The model under review builds one solid part; all positions refer to its coordinate system, in mm. Coordinates: 2 decimals unless noted, no trailing zeros. Order: outer loops, then holes, each group sorted by start corner. A loop starts at its lowest first (then second) coordinate and runs counter-clockwise, first axis right, second up.
```python
from build123d import *

# Parameters (mm, degrees)
BOSS_EXTRUDE1_DEPTH = 2
CUT_EXTRUDE1_DEPTH  = 56.375536238


with BuildPart() as part:
    # Sketch1 → Boss-Extrude1 (new body)
    with BuildSketch(Plane(origin=(0, 0, 0), x_dir=(0, 0, -1), z_dir=(1, 0, 0))):
        with BuildLine():
            Line((0, 9.101653344), (0, 0))
            Line((0, 0), (54, 0))
            Line((54, 0), (54, 1))
            Line((54, 1), (50.535898385, 3))
            Line((50.535898385, 3), (32.535898385, 3))
            Line((32.535898385, 3), (32.535898385, 5))
            Line((32.535898385, 5), (28, 5))
            Line((28, 5), (28, 8.117217781))
            ThreePointArc((28, 8.117217781), (27.749678176, 8.779020345), (27.124034735, 9.109495658))
            Line((27.124034735, 9.109495658), (3.372104204, 12.078486975))
            ThreePointArc((3.372104204, 12.078486975), (1.01459231, 11.350687872), (0, 9.101653344))
        make_face()
        with BuildLine():
            Line((0, 0), (0, -9.101653344))
            ThreePointArc((0, -9.101653344), (1.01459231, -11.350687872), (3.372104204, -12.078486975))
            Line((3.372104204, -12.078486975), (27.124034735, -9.109495658))
            ThreePointArc((27.124034735, -9.109495658), (27.749678176, -8.779020345), (28, -8.117217781))
            Line((28, -8.117217781), (28, -5))
            Line((28, -5), (32.535898385, -5))
            Line((32.535898385, -5), (32.535898385, -3))
            Line((32.535898385, -3), (50.535898385, -3))
            Line((50.535898385, -3), (54, -1))
            Line((54, -1), (54, 0))
            Line((54, 0), (0, 0))
        make_face()
    extrude(amount=BOSS_EXTRUDE1_DEPTH)

    # Sketch2 → Cut-Extrude1 (cut, through all)
    with BuildSketch(Plane(origin=(2, 0, 0), x_dir=(0, 0, -1), z_dir=(1, 0, 0))):
        with BuildLine():
            Line((4.5, -7.578486975), (3.5, -7.578486975))
            ThreePointArc((3.5, -7.578486975), (2.792893219, -7.285593756), (2.5, -6.578486975))
            Line((2.5, -6.578486975), (2.5, 6.421513025))
            ThreePointArc((2.5, 6.421513025), (2.792893219, 7.128619807), (3.5, 7.421513025))
            Line((3.5, 7.421513025), (4.5, 7.421513025))
            ThreePointArc((4.5, 7.421513025), (5.207106781, 7.128619807), (5.5, 6.421513025))
            Line((5.5, 6.421513025), (5.5, -6.578486975))
            ThreePointArc((5.5, -6.578486975), (5.207106781, -7.285593756), (4.5, -7.578486975))
        make_face()
    extrude(amount=-CUT_EXTRUDE1_DEPTH, mode=Mode.SUBTRACT)


solid = part.part
```
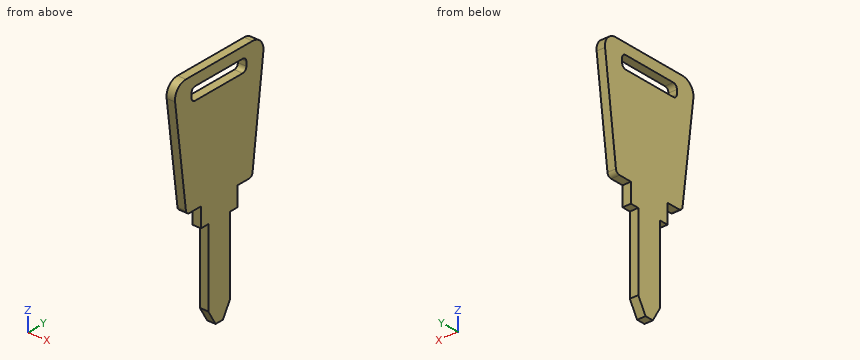
(1) We need section B-B, the plane x = 0.3. Write out the cut boundary in (y, z).
A:
outline: (-12.08, -3.37) - (-9.11, -27.12) arc R1 ccw to (-8.12, -28) - (-5, -28) - (-5, -32.54) - (-3, -32.54) - (-3, -50.54) - (-1, -54) - (1, -54) - (3, -50.54) - (3, -32.54) - (5, -32.54) - (5, -28) - (8.12, -28) arc R1 ccw to (9.11, -27.12) - (12.08, -3.37) arc R3 ccw to (9.1, 0) - (-9.1, 0) arc R3 ccw to start; hole (-7.58, -4.5) arc R1 ccw to (-6.58, -5.5) - (6.42, -5.5) arc R1 ccw to (7.42, -4.5) - (7.42, -3.5) arc R1 ccw to (6.42, -2.5) - (-6.58, -2.5) arc R1 ccw to (-7.58, -3.5) - close
(2) We need section D-D, the plane z = -6. Write out the cut boundary in (x, y).
A:
outline: (0, -11.75) - (2, -11.75) - (2, 11.75) - (0, 11.75) - close
(3) Wall thickness on probe 1 along Z at (x, y) = (1.8, 0); probe 2 along Z at (x, y) = (0.25, -4.25); probe 3 along Y at (x, z) = (1.25, -29): over which ranges is each line inside the solid? List them lowest first.
A:
probe 1: z = -54 to -5.5, -2.5 to 0
probe 2: z = -32.54 to -5.5, -2.5 to 0
probe 3: y = -5 to 5
(4) We need section A-A, the plane y = 4.25. Write out the cut boundary in (x, z), and give its area (3 significant figures).
A:
outline: (0, -32.54) - (2, -32.54) - (2, -5.5) - (0, -5.5) - close; (0, -2.5) - (2, -2.5) - (2, 0) - (0, 0) - close
area: 59.1 mm2
(5) For pin 1 Ø0.6 at (x, y) = (1, 6) entering from -Z; pin 2 Ø0.6 at (x, y) = (1.5, -3) entering from -Z; pin 3 Ø2 at (y, z) = (3.5, -10.5) entering from -X; pin 4 Ø0.6 at (x, z) = (1.5, -38.5) entering from -Y, all flat-tipped, find the tip position at first contact; note any pin that passes through.
A:
pin 1: stops at z = -28
pin 2: stops at z = -51.06
pin 3: stops at x = 0
pin 4: stops at y = -3
(6) We need section C-C, the plane y = 0.5. Write out the cut boundary in (x, z).
A:
outline: (0, -54) - (2, -54) - (2, -5.5) - (0, -5.5) - close; (0, -2.5) - (2, -2.5) - (2, 0) - (0, 0) - close
